Autodesk Inventor part; units mm, degrees
ref_plane "YZ Plane" through (0, 0, 0) normal (1, 0, 0) x (0, 1, 0)
ref_plane "XZ Plane" through (0, 0, 0) normal (0, 1, 0) x (-1, 0, 0)
ref_plane "XY Plane" through (0, 0, 0) normal (0, 0, 1) x (1, 0, 0)
sketch "Sketch1" plane through (0, 0, 0) normal (0, 1, 0) x (-1, 0, 0)
  line L0 (-1.4756, 0) -> (-71.3256, 0)
  line L1 (-71.3256, 0) -> (-71.3256, 165.1)
  line L2 (-71.3256, 165.1) -> (-1.4756, 165.1)
  line L3 (-1.4756, 165.1) -> (-1.4756, 0)
  point P0 (0, 0)
  dimension "d0" = 69.85
  dimension "d1" = 165.1
extrude "Extrusion1" add sketch "Sketch1" along normal blind 3.175
sketch "Sketch3" plane through (0, 0, 0) normal (0, -1, 0) x (1, 0, 0)
  line L0 (71.3256, 165.1) -> (71.3256, 0) construction
  line L1 (71.3256, 0) -> (68.1506, 0) construction
  line L2 (71.3256, 0) -> (1.4756, 0) construction
  line L3 (1.4756, 0) -> (4.6506, 0) construction
  line L4 (68.1506, 0) -> (4.6506, 0)
  line L5 (4.6506, 0) -> (4.6506, 3.175)
  line L6 (4.6506, 3.175) -> (68.1506, 3.175)
  line L7 (68.1506, 3.175) -> (68.1506, 0)
  point P0 (0, 0)
  dimension "d7" = 3.175
  dimension "d8" = 3.175
  dimension "d9" = 63.5
  dimension "d10" = 3.175
extrude "Extrusion3" add sketch "Sketch3" along normal blind 12.7
sketch "Sketch4" plane through (1.4756, 0, 165.1) normal (0, 0, 1) x (1, 0, 0)
  line L0 (69.85, 3.175) -> (0, 3.175)
  line L1 (0, 3.175) -> (69.85, 3.175)
  line L2 (69.85, 3.175) -> (69.85, 0)
  line L3 (69.85, 0) -> (0, 0)
  line L4 (0, 0) -> (0, 3.175)
  point P0 (-1.4756, 0)
extrude "Extrusion4" add sketch "Sketch4" along normal blind 17.78
properties part number "False_Bottom_2"
Work out the finished part from the listing and answer in its coordinate system (mm). A direction names the side the tool comes from. Round coordinates to 2 decimals unless told otherwise and drop trailing zeros. Loops run counter-clockwise (first coordinate to the right, second up) from the corner with the lowest first, then second, coordinate; pieces in that order, holes last. Notation, with made-up numbers: M 9,-15.5 L 48,-15.5 A20 ccw 48,20.5 Z; hole C 27.5,46.25 d6. An arc over 180 degrees is marked long. Use CSV: the item, a comma, the result in double quotes.
Q1. Section C-C, the plane y = -2.5 is taken. Determine the outline of the cut face in (x, z) (3 decimals).
Determined:
outline,"M 4.651,0 L 68.151,0 L 68.151,3.175 L 4.651,3.175 Z"
Q2. A tool of negligible diameter and unlimited length cuts with its end or side. For faces 1 (the flat face through (4.651, -6, 2)), 2 (the flat face through (36, -6, 3.175)), 3 (the flat face through (68.151, -6, 2)), from which of +Z, -Z, +X, -X, +Y, -Y can it reach the whole face along a straight path? Write none if from no direction.
Determined:
face 1,"+Z, -Z, -X, -Y"
face 2,"+Z, +X, -X, -Y"
face 3,"+Z, -Z, +X, -Y"
Q3. Section A-A, the plane x = 50.5 is taken. Determine the outline of the cut face in (y, z) (3 decimals).
Determined:
outline,"M -12.7,0 L 3.175,0 L 3.175,182.88 L 0,182.88 L 0,3.175 L -12.7,3.175 Z"
Q4. Section B-B, the plane z = 54 is taken. Determine the outline of the cut face in (x, y) (3 decimals).
Determined:
outline,"M 1.476,0 L 71.326,0 L 71.326,3.175 L 1.476,3.175 Z"
Q5. Each of these flat-tipped pins is pushed along its axis until it touches: pin 1 (3.5 mm diameter, centred on y = -5.5, z = 1.5, fed in from -X); pin 2 (3.5 mm diameter, centred on y = -6.5, z = 1, fed in from +X); pin 3 (21 mm diameter, centred on x = 31, z = 90.5, fed in from -Y). Where does it stop, or does it pass through?
Determined:
pin 1,"x = 4.65"
pin 2,"x = 68.15"
pin 3,"y = 0"
Q6. Consider L1, parallel to Z at x = 11.5, y = -5.25 (3 decimals). Determine where the line is inside the solid, lowest interval first.
Determined:
L1,"0 to 3.175"
